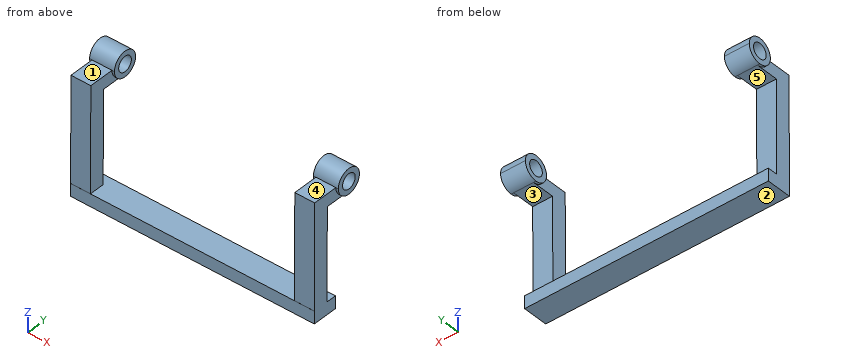
from build123d import *

# Parameters (mm, degrees)
F1_DEPTH      = 6.35
F1_DEPTH_BACK = 6.35
F2_DEPTH      = 5.08
F2_DEPTH_BACK = 5.08
F6_DEPTH      = 120.14245


with BuildPart() as f1:
    # F0 (on Right) → F1 (new body, two sides)
    with BuildSketch(Plane.YZ) as f1_sk:
        with BuildLine():
            ThreePointArc((6.35, 0), (0, 6.35), (-6.35, 0))
            ThreePointArc((-6.35, 0), (-4.490128, -4.490128), (0, -6.35))
            ThreePointArc((0, -6.35), (4.490128, -4.490128), (6.35, 0))
        make_face()
        with BuildLine():
            ThreePointArc((-3.81, 0), (0, 3.81), (3.81, 0))
            ThreePointArc((3.81, 0), (0, -3.81), (-3.81, 0))
        make_face(mode=Mode.SUBTRACT)
    extrude(amount=F1_DEPTH)
    extrude(f1_sk.sketch, amount=-F1_DEPTH_BACK)

    # F0 (on Right) → F2 (join, two sides)
    with BuildSketch(Plane.YZ) as f2_sk:
        with BuildLine():
            ThreePointArc((0, -6.35), (-4.490128, -4.490128), (-6.35, 0))
            Line((-6.35, 0), (-19.05, 0))
            Line((-19.05, 0), (-19.264068, -53.31585))
            Line((-19.264068, -53.31585), (-11.644068, -53.31585))
            Line((-11.644068, -53.31585), (-11.455496, -6.35))
            Line((-11.455496, -6.35), (0, -6.35))
        make_face()
        Polygon((-19.289564, -59.66585), (-19.264068, -53.31585), (-19.289564, -53.31585), align=None)
        Polygon((-11.644068, -53.31585), (-19.264068, -53.31585), (-19.289564, -59.66585), (-11.669564, -59.66585), align=None)
        Polygon((-6.589564, -53.31585), (-11.644068, -53.31585), (-11.669564, -59.66585), (-6.589564, -59.66585), align=None)
    extrude(amount=F2_DEPTH)
    extrude(f2_sk.sketch, amount=-F2_DEPTH_BACK)



with BuildPart() as f4_1:
    # F4: instance of F1
    add(f1.part.mirror(Plane.YZ.offset(-57.15)))


with BuildPart() as f1_1:
    add(f1.part)

    add(f4_1.part)  # F6 merges F4_1
    # F5 (on face) → F6 (join)
    with BuildSketch(Plane.YZ.offset(5.08)):
        Polygon((-11.644068, -53.31585), (-19.264068, -53.31585), (-19.289564, -53.31585), (-19.289564, -59.66585), (-6.589564, -59.66585), (-6.589564, -53.31585), align=None)
    extrude(amount=-F6_DEPTH)


solid = f1_1.part
Can you work these out from the model? Positions are in its coordinate system, mm. Face numbers are marked on the shaded views. A direction names the side the tool comes from. Give positions to 0.01 mm unless a question says otherwise; leave off trailing zeros. Loops run counter-clockwise (first coordinate to the right, second up) from the corner with the lowest first, then second, coordinate; pieces in that order, holes last. Notation, with made-up numbers: M 40.5,-1 L 73.5,-1 A22 ccw 73.5,17 Z; hole C 55,84.5 d1. An arc over 180 degrees is marked long. One line per item, written item: value. Start each with the question number.
1) If we section it at A-A, the plane z = -39: Write out the boundary of the cut face in (x, y), and give its area (3 significant figures).
2) If we section it at B-B, the plane x = -13.5: Write out the boundary of the cut face in (y, z).
3) Thinking about a two-plate mould opening in Z: for the marked faces 1, 2 and 3, which applies, +Z half, -Z half, draft (parallel to the pull), parting line (faces both ways), or undercut?
4) I'm going to push flat-ended pins straight in: pin 1 (4 mm diameter, centred on x = -83.5, y = -13, fed in from +Z); pin 2 (3 mm diameter, centred on x = 1, y = -10, fed in from +Z); pin 3 (9.5 mm diameter, centred on y = -11, z = -36.5, fed in from -X). Where does each tip first touch, or does it pass through?
5) On a 3-axis mill with a long thin cutter (end or side, diameter ignored), from which of +Z, -Z, +X, -X, +Y, -Y can I reach the whole of each face in a straight line? I mean the marked faces 4 and 5. Say none if no direction works.
6) If I drill on line 1 (Z direction, x = -3.25, y = 0); line 2 (X direction, y = -8, z = -1.5); line 3 (Z direction, x = -79.5, y = -13.75), over which ranges is the centre line in solid material (lowest first)? Write a range as [from, to].
Completed:
1. outline: M -119.38,-19.21 L -109.22,-19.21 L -109.22,-11.59 L -119.38,-11.59 Z; M -5.08,-19.21 L 5.08,-19.21 L 5.08,-11.59 L -5.08,-11.59 Z
1. area: 155 mm^2
2. outline: M -19.29,-59.67 L -6.59,-59.67 L -6.59,-53.32 L -19.29,-53.32 Z
3. face 1: +Z half
3. face 2: -Z half
3. face 3: undercut
4. pin 1: stops at z = -53.32
4. pin 2: stops at z = 0
4. pin 3: stops at x = -119.38
5. face 4: +Z, +X, -X, -Y
5. face 5: +X, -X, +Y
6. line 1: z = [-6.35, -3.81], [3.81, 6.35]
6. line 2: x = [-119.38, -109.22], [-5.08, 5.08]
6. line 3: z = [-59.67, -53.32]
